from build123d import *

# Parameters (mm, degrees)
EXTRUDE2_DEPTH                 = 26
CUT_EXTRUDE3_DEPTH             = 28.147743921
CHAMFER1_SIZE                  = 1
CHAMFER2_SIZE2                 = 1.154700538
CHAMFER2_SIZE                  = 2
CHAMFER3_SIZE2                 = 1.154700538
CHAMFER3_SIZE                  = 2
CHAMFER4_SIZE                  = 1.5
CHAMFER4_SIZE2                 = 0.866025404
CUT_EXTRUDE5_REACH             = 29.148
CUT_EXTRUDE5_DIRECTION_2_REACH = 29.148
CUT_EXTRUDE6_START             = 4.5
CUT_EXTRUDE6_DEPTH             = 10.5
CUT_EXTRUDE6_START_2           = 15
CUT_EXTRUDE6_2_DEPTH           = 3
CUT_EXTRUDE6_START_3           = -4
CUT_EXTRUDE6_3_DEPTH           = 8


with BuildPart() as part:
    # Sketch1 → Extrude2 (new body)
    with BuildSketch(Plane.XY):
        Polygon((-5, 0), (5, 0), (5, 6), (2, 6), (2, 3), (-2, 3), (-2, 6), (-5, 6), align=None)
    extrude(amount=EXTRUDE2_DEPTH)

    # Sketch2 → Cut-Extrude3 (cut, through all)
    with BuildSketch(Plane(origin=(0, 0, 0), x_dir=(1, 0, 0), z_dir=(0, 1, 0))):
        with BuildLine():
            Line((-5, 1), (5, 1))
            Line((5, 1), (5, -5))
            ThreePointArc((5, -5), (0, 0), (-5, -5))
            Line((-5, -5), (-5, 1))
        make_face()
    extrude(amount=CUT_EXTRUDE3_DEPTH, mode=Mode.SUBTRACT)

    # Chamfer1
    chamfer1_edges = [part.edges().sort_by_distance(p)[0] for p in [
        (5, 0, 15.5),
        (-5, 0, 15.5),
        (0, 0, 0),
    ]]
    chamfer(chamfer1_edges, length=CHAMFER1_SIZE)

    # Chamfer2
    chamfer2_edges = [part.edges().sort_by_distance(p)[0] for p in [
        (5, 6, 15.5),
        (4.183300133, 6, 2.261387212),
    ]]
    chamfer(chamfer2_edges, length=CHAMFER2_SIZE, length2=CHAMFER2_SIZE2)

    # Chamfer3
    chamfer3_edges = [part.edges().sort_by_distance(p)[0] for p in [
        (-5, 6, 15.5),
        (-4.183300133, 6, 2.261387212),
    ]]
    chamfer(chamfer3_edges, length=CHAMFER3_SIZE, length2=CHAMFER3_SIZE2)

    # Chamfer4
    chamfer4_edges = [part.edges().sort_by_distance(p)[0] for p in [
        (0, 3, 0),
    ]]
    chamfer4_side = [part.faces().sort_by_distance(p)[0] for p in [
        (0, 3, 13.068070345),
    ]]
    chamfer(chamfer4_edges, length=CHAMFER4_SIZE, length2=CHAMFER4_SIZE2, reference=chamfer4_side[0])

    # Cut-Extrude5: up to this face of the body (flat: up to its plane)
    cut_extrude5_end = Plane(part.part.faces().sort_by_distance((-2, 4.468849855, 13.300187557))[0])
    # Sketch5 → Cut-Extrude5 (cut, up to the picked face)
    with BuildSketch(Plane(origin=(0, 0, 0), x_dir=(0, 0, -1), z_dir=(1, 0, 0)), mode=Mode.PRIVATE) as cut_extrude5_sk1:
        with BuildLine():
            Line((-15, 3), (-14, 3))
            Line((-14, 3), (-14, 0))
            Line((-14, 0), (-18, 0))
            ThreePointArc((-18, 0), (-15.878679656, 0.878679656), (-15, 3))
        make_face()
    cut_extrude5_tool1 = split(extrude(cut_extrude5_sk1.sketch, amount=-CUT_EXTRUDE5_REACH, mode=Mode.PRIVATE), bisect_by=cut_extrude5_end, keep=Keep.BOTH, mode=Mode.PRIVATE)
    add(cut_extrude5_tool1.solids().sort_by(Axis((0, 1.174967, 14.958278), (-1, 0, 0)))[0], mode=Mode.SUBTRACT)

    # Cut-Extrude5 direction 2: up to this face of the body (flat: up to its plane)
    cut_extrude5_direction_2_end = Plane(part.part.faces().sort_by_distance((2, 4.468849855, 13.300187557))[0])
    # Sketch5 → Cut-Extrude5 direction 2 (cut, up to the picked face)
    with BuildSketch(Plane(origin=(0, 0, 0), x_dir=(0, 0, -1), z_dir=(1, 0, 0)), mode=Mode.PRIVATE) as cut_extrude5_direction_2_sk1:
        with BuildLine():
            Line((-15, 3), (-14, 3))
            Line((-14, 3), (-14, 0))
            Line((-14, 0), (-18, 0))
            ThreePointArc((-18, 0), (-15.878679656, 0.878679656), (-15, 3))
        make_face()
    cut_extrude5_direction_2_tool1 = split(extrude(cut_extrude5_direction_2_sk1.sketch, amount=CUT_EXTRUDE5_DIRECTION_2_REACH, mode=Mode.PRIVATE), bisect_by=cut_extrude5_direction_2_end, keep=Keep.BOTH, mode=Mode.PRIVATE)
    add(cut_extrude5_direction_2_tool1.solids().sort_by(Axis((0, 1.174967, 14.958278), (1, 0, 0)))[0], mode=Mode.SUBTRACT)

    # Cut-Extrude6: read off the stored shape, not the designer's step
    # Cut-Extrude6 outline → Cut-Extrude6 (cut)
    with BuildSketch(Plane.XY.offset(CUT_EXTRUDE6_START)):
        Polygon((-2, 3), (-4, 0), (4, 0), (2, 3), align=None)
    extrude(amount=CUT_EXTRUDE6_DEPTH, mode=Mode.SUBTRACT)

    # Cut-Extrude6 2 outline → Cut-Extrude6 2 (cut)
    with BuildSketch(Plane.XY.offset(CUT_EXTRUDE6_START_2)):
        Polygon((2, 3), (2, 0), (4, 0), align=None)
        Polygon((-2, 3), (-4, 0), (-2, 0), align=None)
    extrude(amount=CUT_EXTRUDE6_2_DEPTH, mode=Mode.SUBTRACT)

    # Cut-Extrude6 3 outline → Cut-Extrude6 3 (add)
    with BuildSketch(Plane.YZ.offset(CUT_EXTRUDE6_START_3)):
        with BuildLine():
            ThreePointArc((0, 18), (0.878679656, 15.878679656), (3, 15))
            Line((3, 15), (3, 18))
            Line((3, 18), (0, 18))
        make_face()
    extrude(amount=CUT_EXTRUDE6_3_DEPTH)


solid = part.part
Verification items for the finished model (mm, model axes). A direction names the side the tool comes from. Round coordinates to 2 decimals unless told otherwise and drop trailing zeros. Loops run counter-clockwise (first coordinate to the right, second up) from the corner with the lowest first, then second, coordinate; pieces in that order, holes last. Notation, with made-up numbers: M 32,-26.75 L 82,-26.75 A18 cw 82,-2.75 Z; hole C 87.5,42 d9. An arc over 180 degrees is marked long. Write each question's results on one line, items separated by ' | '.
1) Scan lines: L1, parallel to X at y = 5.75, z = 22.25; L2, parallel to X at y = 3.5, z = 18.5; L3, parallel to Y at x = 1.75, z = 2.75. Record each from-to range of solid material in increasing order. Write a range as from..to.
Checks:
L1: x = -3.99..-2, 2..3.99 | L2: x = -5..-2, 2..5 | L3: y = 0..3
2) Section check C-C on x = 0. Record the boundary of the cut face in (y, z).
Checks:
outline: M 0,1 L 1,0 L 2.13,0 L 3,1.5 L 3,4.5 L 0,4.5 Z; M 0,18 A3 ccw 3,15 L 3,26 L 0,26 Z
3) Section check A-A on y = 3.5. Record the boundary of the cut face in (x, z), then the cut area to 3 significant figures.
Checks:
outline: M -5,5 A5 ccw -2,0.42 L -2,26 L -5,26 Z; M 2,0.42 A5 ccw 5,5 L 5,26 L 2,26 Z | area: 146 mm2
4) Access from +Z, -Z, +X, -X, +Y, -Y to the whole of each face (thin tool, end or side, straight path). Record for faces 1 (the flat face through (0, 3, 20)), 2 (the flat face through (-3, 1.5, 9.7)), 3 (the flat face through (-4.5, 0.5, 15.6)).
Checks:
face 1: +Z, -Z, +Y | face 2: -Y | face 3: +Z, -Z, -X, -Y
5) Section check B-B on z = 7.5. Record the boundary of the cut face in (x, y).
Checks:
outline: M -5,1 L -4,0 L -2,3 L -2,6 L -3.85,6 L -5,4 Z; M 2,3 L 4,0 L 5,1 L 5,4 L 3.85,6 L 2,6 Z
6) Mould release check, pull along X, two halves, no side actions. Record for faces 4 (the cylindrical face through (-0.06, 0.52, 16.31)), 5 (the flat face through (0, 0, 3)), 6 (the flat face through (-4.415, 5.014, 15.353)): released by +X, released by -X, zero draft, split by the parting line, or undercut.
Checks:
face 4: undercut | face 5: zero draft | face 6: released by -X
7) Gauge pin test, flat ends, axial feed: P1, Ø1.5, axis at x = -0.5, z = 3.5, coming from the +Y side; P2, Ø4.5, axis at x = -0.5, z = 20.5, coming from the +Y side. Record the tip position at first contact, or that the pin passes through.
Checks:
P1: stops at y = 3 | P2: stops at y = 6
8) Section check D-D on z = 24.25. Record the boundary of the cut face in (x, y), then the cut area to 3 significant figures.
Checks:
outline: M -5,1 L -4,0 L 4,0 L 5,1 L 5,4 L 3.85,6 L 2,6 L 2,3 L -2,3 L -2,6 L -3.85,6 L -5,4 Z | area: 44.7 mm2
